Verification items for the finished model (mm, model axes). Face numbers are marked on the shaded views. A direction names the side the tool comes from. Coordinates: 2 decimals unless noted, no trailing zeros. Write each loop counter-clockwise with the first axis right and the second up, starting at its lowest first coordinate (ties: lowest second). Pieces come first, ordered by that corner, then holes. Notation, with made-up numbers: M 44,55.5 L 93,55.5 A9 ccw 93,71.5 Z; hole C -6.5,-19 d6. An arc over 180 degrees is marked long. Answer in a Markdown table with one row per item.
Autodesk Inventor part; units mm, degrees
ref_plane "YZ Plane" through (0, 0, 0) normal (1, 0, 0) x (0, 1, 0)
ref_plane "XZ Plane" through (0, 0, 0) normal (0, 1, 0) x (-1, 0, 0)
ref_plane "XY Plane" through (0, 0, 0) normal (0, 0, 1) x (1, 0, 0)
sketch "Sketch1" plane through (0, 0, 0) normal (0, 1, 0) x (-1, 0, 0)
  line L0 (-42.0064, -29.8829) -> (-42.0064, 29.6171)
  line L1 (-42.0064, 29.6171) -> (42.9936, 29.6171)
  line L2 (42.9936, 29.6171) -> (42.9936, -29.8829)
  line L3 (42.9936, -29.8829) -> (-42.0064, -29.8829)
  circle A0 centre (-36.5064, 24.1171) radius 1.6
  circle A1 centre (-36.5064, -24.3829) radius 1.6
  circle A2 centre (37.4936, -24.3829) radius 1.6
  circle A3 centre (37.4936, 24.1171) radius 1.6
  line L4 (-42.5064, -29.8829) -> (-42.5064, 30.1171)
  line L5 (-42.5064, 30.1171) -> (43.4936, 30.1171)
  line L6 (43.4936, -29.8829) -> (43.4936, 30.1171)
  line L7 (-42.5064, -30.3829) -> (43.4936, -30.3829)
  line L8 (-42.5064, -29.8829) -> (-42.5064, -30.3829)
  line L9 (43.4936, -30.3829) -> (43.4936, -29.8829)
  line L10 (-44.5064, -32.3829) -> (45.4936, -32.3829)
  line L11 (45.4936, -32.3829) -> (45.4936, 32.1171)
  line L12 (45.4936, 32.1171) -> (-44.5064, 32.1171)
  line L13 (-44.5064, 32.1171) -> (-44.5064, -32.3829)
  point P0 (0, 0)
  dimension "d0" = 0.5
  dimension "d1" = 0.5
  dimension "d2" = 0.5
  dimension "d3" = 0.5
  dimension "d4" = 2
  dimension "d5" = 2
  dimension "d6" = 2
  dimension "d7" = 2
extrude "Extrusion1" add sketch "Sketch1" along normal blind 25 contours L13 L12 L11 L10
extrude "Extrusion2" add sketch "Sketch1" along normal blind 2 contours L0 L1 L2 L3 | L4 L5 L6 L9 L7 L8
fillet "Fillet1" radius 3 4 edges at (44.5064, 12.5, 32.1171) (44.5064, 12.5, -32.3829) (-45.4936, 12.5, -32.3829) (-45.4936, 12.5, 32.1171)
fillet "Fillet2" radius 1 8 edges at (43.6277, 0, 31.2384) (44.5064, 0, -0.1329) (43.6277, 0, -31.5042) (-0.4936, 0, -32.3829) (-44.615, 0, -31.5042) (-45.4936, 0, -0.1329) (-44.615, 0, 31.2384) (-0.4936, 0, 32.1171)
chamfer "Chamfer1" distance 0.5 angle 45 8 edges at (-0.4936, 25, 32.1171) (43.6277, 25, 31.2384) (44.5064, 25, -0.1329) (43.6277, 25, -31.5042) (-0.4936, 25, -32.3829) (-44.615, 25, -31.5042) (-45.4936, 25, -0.1329) (-44.615, 25, 31.2384)
fillet "Fillet3" radius 0.5 1 edges at (42.5064, 13.5, 30.1171)
fillet "Fillet4" radius 0.5 1 edges at (42.5064, 13.5, -30.3829)
fillet "Fillet5" radius 0.5 1 edges at (-43.4936, 13.5, -30.3829)
fillet "Fillet6" radius 0.5 1 edges at (-43.4936, 13.5, 30.1171)
sketch "Sketch2" plane through (0, 2, 0) normal (0, 1, 0) x (1, 0, 0)
  circle A0 centre (36.5064, -24.1171) radius 1.6
  circle A1 centre (-37.4936, -24.1171) radius 1.6
  circle A2 centre (-37.4936, 24.3829) radius 1.6
  circle A3 centre (36.5064, 24.3829) radius 1.6
  circle A4 centre (36.5064, -24.1171) radius 3
  circle A5 centre (-37.4936, -24.1171) radius 3
  circle A6 centre (-37.4936, 24.3829) radius 3
  circle A7 centre (36.5064, 24.3829) radius 3
  point P0 (0, 0)
  dimension "d21" = 6
  dimension "d22" = 6
  dimension "d23" = 6
  dimension "d24" = 6
extrude "Extrusion3" add sketch "Sketch2" along normal blind 2
sketch "Sketch3" plane through (41.5064, 1, -32.3829) normal (0, 0, -1) x (-1, 0, 0)
  point P0 (41.5064, -1)
sketch "Sketch4" plane through (-45.4936, 1, -29.3829) normal (-1, 0, 0) x (0, 0, 1)
  line L0 (49.3829, 17.5) -> (9.3829, 17.5) construction
  line L1 (49.3829, 13.5) -> (9.3829, 13.5)
  line L2 (9.3829, 21.5) -> (49.3829, 21.5)
  arc A0 (49.3829, 13.5) -> (49.3829, 21.5) centre (49.3829, 17.5) ccw
  arc A1 (9.3829, 21.5) -> (9.3829, 13.5) centre (9.3829, 17.5) ccw
  line L3 (0, 23.5) -> (58.5, 23.5)
  line L4 (5.3829, 17.5) -> (5.3829, 24)
  line L5 (53.3829, 17.5) -> (53.3829, 24)
  line L6 (59, 24) -> (-0.5, 24)
  line L7 (5.3829, 24) -> (53.3829, 24)
  line L8 (61.5, 0) -> (61.5, 23.5)
  line L9 (29.3829, -1) -> (29.3829, 24)
  point P0 (29.3829, 17.5)
  point P1 (5.3829, 24)
  point P2 (29.3829, 11.5)
  dimension "d27" = 2
  dimension "d28" = 8
  dimension "d38" = 48
  dimension "d39" = 0
extrude "Extrusion4" cut sketch "Sketch4" against normal blind 200 contours L1 L9 L2 A0 | L1 A1 L2 L9
extrude "Extrusion5" cut sketch "Sketch4" against normal blind 200 contours A0 L2 L9 L3 L5 | L2 A1 L4 L3 L9 | L3 L9 L6 L5 | L3 L4 L6 L9
sketch "Sketch5" plane through (41.5064, 1, -32.3829) normal (0, 0, -1) x (-1, 0, 0)
  line L0 (73, 7.5) -> (63, 7.5) construction
  line L1 (73, 11.5) -> (63, 11.5)
  line L2 (63, 3.5) -> (73, 3.5)
  arc A0 (73, 3.5) -> (73, 11.5) centre (73, 7.5) ccw
  arc A1 (63, 11.5) -> (63, 3.5) centre (63, 7.5) ccw
  line L3 (41.5064, -1) -> (41.5064, 23.5)
  line L4 (0, 23.5) -> (84, 23.5)
  line L5 (10.0127, 7.5) -> (20.0127, 7.5) construction
  line L6 (10.0127, 11.5) -> (20.0127, 11.5)
  line L7 (20.0127, 3.5) -> (10.0127, 3.5)
  arc A2 (10.0127, 11.5) -> (10.0127, 3.5) centre (10.0127, 7.5) ccw
  arc A3 (20.0127, 3.5) -> (20.0127, 11.5) centre (20.0127, 7.5) ccw
  line L8 (0, -1) -> (84, -1)
  line L9 (6.0127, 7.5) -> (6.0127, 24)
  line L10 (84.5, 24) -> (-0.5, 24)
  line L11 (24.0127, 7.5) -> (24.0127, 24)
  line L12 (6.0127, 24) -> (24.0127, 24)
  line L13 (59, 7.5) -> (59, 24)
  line L14 (77, 7.5) -> (77, 24)
  line L15 (59, 24) -> (77, 24)
  line L16 (59, 24) -> (59, 15.5271)
  line L17 (59, 15.5271) -> (77, 15.5271)
  line L18 (77, 15.5271) -> (77, 24)
  line L19 (6.0127, 24) -> (24.0127, 24)
  line L20 (59, 24) -> (77, 24)
  line L21 (68, 7.5) -> (68, 24) construction
  line L22 (15.0127, 7.5) -> (15.0127, 24) construction
  line L23 (84, 23.5) -> (84, 0)
  point P0 (84, 11.75)
  dimension "d40" = 5
  dimension "d41" = 8
  dimension "d42" = 4.5
  dimension "d45" = 7
extrude "Extrusion6" cut sketch "Sketch5" against normal blind 200 contours A0 L2 A1 L1 | L1 A1 L13 L17 L14 A0 | L17 L13 L4 L14 | L4 L13 L10 L14 | L11 A3 L6 A2 L9 L4 | L4 L9 L10 L11 | A3 L7 A2 L6
sketch "Sketch6" plane through (-42.4936, 1, 32.1171) normal (0, 0, 1) x (1, 0, 0)
  line L0 (46.1174, 12.771) -> (38.8698, 12.771) construction
  line L1 (46.1174, 11) -> (38.8698, 11)
  line L2 (38.8698, 14.5419) -> (46.1174, 14.5419)
  arc A0 (46.1174, 11) -> (46.1174, 14.5419) centre (46.1174, 12.771) ccw
  arc A1 (38.8698, 14.5419) -> (38.8698, 11) centre (38.8698, 12.771) ccw
  line L3 (37.0989, 12.771) -> (37.0989, 32.771)
  line L4 (37.0989, 32.771) -> (47.8884, 32.771)
  line L5 (47.8884, 32.771) -> (47.8884, 12.771)
  arc A2 (21, 3.5) -> (25, 7.5) centre (21, 7.5) ccw
  line L6 (84.5, 1) -> (-0.5, 1)
  point P0 (42.4936, -1)
  point P1 (42.4936, 12.771)
  point P2 (42.4936, 11)
  point P3 (42.4936, 14.5419)
  dimension "d46" = 3.5419
  dimension "d50" = 20
  dimension "d51" = 10
extrude "Extrusion7" cut sketch "Sketch6" against normal blind 15
properties part number "cutie_3DPrint"
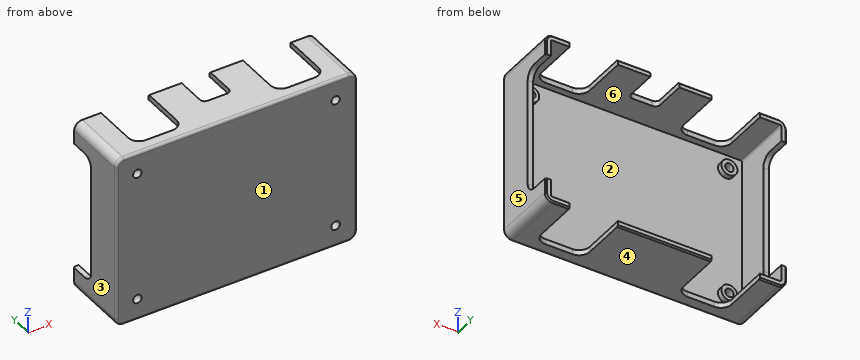
1) Sectioned sample at C-C (z = 11). Record the cut outline in (x, y).
Response values:
| item | result |
|---|---|
| outline | M -45.49,1 A1 ccw -44.49,0 L 43.51,0 A1 ccw 44.51,1 L 44.51,14.5 L 42.51,14.5 L 42.51,2 L -43.49,2 L -43.49,14.5 L -45.49,14.5 Z |
2) Sectioned sample at A-A (x = 30). Record the cut outline in (y, z), then the cut area to 3 significant figures.
Response values:
| item | result |
|---|---|
| outline | M 0,-31.38 A1 ccw 1,-32.38 L 4.5,-32.38 L 4.5,-30.38 L 2,-30.38 L 2,30.12 L 4.5,30.12 L 4.5,32.12 L 1,32.12 A1 ccw 0,31.12 Z |
| area | 139 mm² |
3) Sectioned sample at B-B (x = -37). Record the cut outline in (y, z).
Response values:
| item | result |
|---|---|
| outline | M 0,-31.38 A1 ccw 1,-32.38 L 24.5,-32.38 L 25,-31.88 L 25,-30.38 L 2,-30.38 L 2,-27.34 L 4,-27.34 L 4,-25.9 L 0,-25.9 Z; M 0,-22.86 L 4,-22.86 L 4,-21.42 L 2,-21.42 L 2,21.16 L 4,21.16 L 4,22.6 L 0,22.6 Z; M 0,25.64 L 4,25.64 L 4,27.08 L 2,27.08 L 2,30.12 L 25,30.12 L 25,31.62 L 24.5,32.12 L 1,32.12 A1 ccw 0,31.12 Z |
4) Tool access check on the marked faces 1 and 2. Record the directions out of +Z, -Z, +X, -X, +Y, -Y that give a thin tool (end or side, any length) a straight path to the whole face; none if there is none.
Response values:
| item | result |
|---|---|
| face 1 | +Z, -Z, +X, -X, -Y |
| face 2 | +Y |
5) Release check for a two-part mould opening along X. For the marked faces 3, 4, 5 and 6 record: +X half, -X half, draft (parallel to the pull), parting line (faces both ways), or undercut.
Response values:
| item | result |
|---|---|
| face 3 | -X half |
| face 4 | draft |
| face 5 | +X half |
| face 6 | undercut |
6) Sectioned sample at D-D (y = 17.25). Give the number of separate pieces and of enclosed holes in the cut face, then the cut area to 3 significant figures.
Response values:
| item | result |
|---|---|
| separate pieces | 7 |
| enclosed holes | 0 |
| area | 239 mm² |
7) Depth check by flat-ended pin: pin 1 (1.8 mm diameter, centred on x = 35, z = 24.5, fed in from +Y); pin 2 (2 mm diameter, centred on x = -26, z = 30.5, fed in from +Y); pin 3 (1 mm diameter, centred on x = 0, z = 31.5, fed in from +Y); pin 4 (7 mm diameter, centred on x = 19.5, y = 18.5, fed in from -Z). Enter the tip coordinate at first touch or a pass-through.
Response values:
| item | result |
|---|---|
| pin 1 | stops at y = 4 |
| pin 2 | stops at y = 4.5 |
| pin 3 | stops at y = 12 |
| pin 4 | stops at z = -32.38 |
8) Thickness scan on L1, parallel to Z at x = 9.5, y = 6.25; L2, parallel to X at y = 11, z = -16; L3, parallel to Y at x = 6, z = -8. Record the ranges inside material, lowest first. Write a range as [from, to].
Response values:
| item | result |
|---|---|
| L1 | z = [-32.38, -30.38], [30.12, 32.12] |
| L2 | x = [-45.49, -43.49], [42.51, 44.51] |
| L3 | y = [0, 2] |
